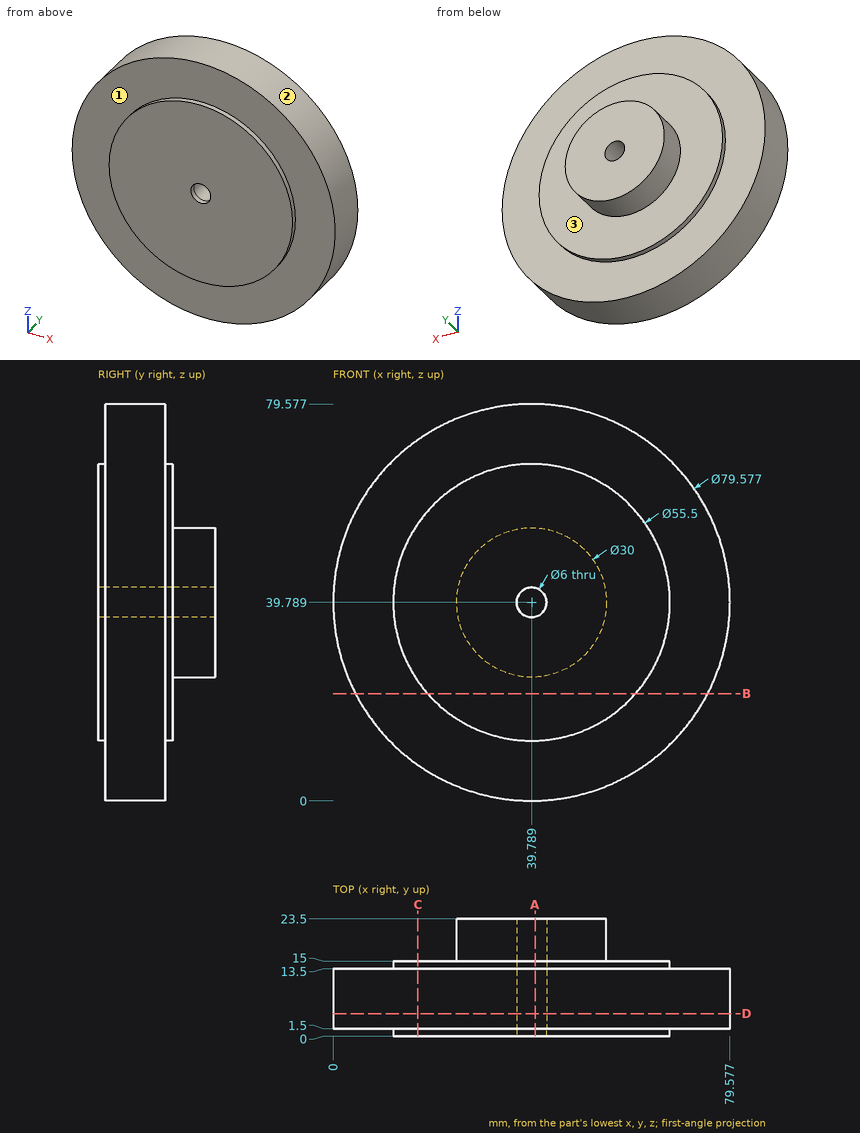
Check sheet for the drawn part. Datum: minimum x, y, z corner. Units: mm. A direction names the side the tool comes from. Give positions to 0.01 mm unless a question says otherwise; leave off trailing zeros. Write each loop counter-clockwise with the first axis right and the second up, starting at its lowest first coordinate (ties: lowest second). Pieces come first, ordered by that corner, then holes.
(1) Cross-section at A-A (x = 40.5). Enter the section's corners in (y, z) (1 decimal).
(2) Cross-section at B-B (z = 21.5). Enter the section's corners in (x, y) (1 decimal).
(3) Cross-section at D-D (y = 4.5). Enter the section's corners in (x, z), plus the area to 3 significant figures.
(4) Cross-section at C-C (x = 17). Enter the section's corners in (y, z) (1 decimal).
(5) Gauge pin test, flat ends, axial feed: pin 1 (3 mm diameter, centred on x = 14.5, z = 16, fed in from +Y); pin 2 (6 mm diameter, centred on x = 65.5, z = 31, fed in from +Y); pin 3 (2 mm diameter, centred on y = 5.5, z = 28.5, fed in from +X) (1 decimal). Record the tip position at first contact, or that the pin passes through.
(6) Access from +Z, -Z, +X, -X, +Y, -Y to the whole of each face (thin tool, end or side, straight path). Record for the marked faces 1, 2 and 3.
(7) Material ranges on line 1 (Y direction, x = 14.5, z = 62); line 2 (Y direction, x = 51, z = 54.5); line 3 (X direction, y = 18.75, z = 36) (1 decimal), recorded low to high.
Worked out:
1. outline: (0, 12) - (1.5, 12) - (1.5, 0) - (13.5, 0) - (13.5, 12) - (15, 12) - (15, 24.8) - (23.5, 24.8) - (23.5, 36.9) - (0, 36.9) - close; (0, 42.7) - (23.5, 42.7) - (23.5, 54.8) - (15, 54.8) - (15, 67.5) - (13.5, 67.5) - (13.5, 79.6) - (1.5, 79.6) - (1.5, 67.5) - (0, 67.5) - close
2. outline: (4.5, 1.5) - (18.9, 1.5) - (18.9, 0) - (60.7, 0) - (60.7, 1.5) - (75.1, 1.5) - (75.1, 13.5) - (60.7, 13.5) - (60.7, 15) - (18.9, 15) - (18.9, 13.5) - (4.5, 13.5) - close
3. outline: circle Ø79.58 at (39.79, 39.79); hole circle Ø6 at (39.79, 39.79)
3. area: 4,950 mm2
4. outline: (0, 24) - (1.5, 24) - (1.5, 7.2) - (13.5, 7.2) - (13.5, 24) - (15, 24) - (15, 55.6) - (13.5, 55.6) - (13.5, 72.4) - (1.5, 72.4) - (1.5, 55.6) - (0, 55.6) - close
5. pin 1: stops at y = 13.5
5. pin 2: stops at y = 15
5. pin 3: stops at x = 78.2
6. face 1: -Y
6. face 2: +Y, -Y
6. face 3: +Y
7. line 1: y = 1.5 to 13.5
7. line 2: y = 0 to 15
7. line 3: x = 25.3 to 54.3
